Source: three-view drawing plus pictorial views. Frame: mm from the lowest corner of the part. Round coordinates to 2 decimals unless told otherwise and drop trailing zeros. Loops run counter-clockwise (first coordinate to the right, second up) from the corner with the lowest first, then second, coordinate; pieces in that order, holes last. Notation, with made-up numbers: (6, -5) -> (15, -5) arc R8 cw to (15, 8) -> close; hole circle Ø1 at (89, 20). An arc over 180 degrees is marked (long way). Put each result on its own line as item: value. Start each with the question number.
1. Cut plane B-B (y = 52.5). Return the cut outline in (x, z).
2. Cut plane C-C (z = 3.3). State how many separate pieces and enclosed holes the cut face has, then the cut area to 3 significant figures.
3. Cut plane D-D (y = 43). Return the cut outline in (x, z), then the cut area to 3 significant figures.
4. Material intervals for L1, parallel to X at y = 59, z = 1.5; L2, parallel to X at y = 62.5, z = 2.25; L3, parallel to Y at x = 12, z = 1.75, sorted ascending.
5. Cut plane A-A (x = 12). Return the cut outline in (y, z), then the cut area to 3 significant figures.
6. Contact query for flat-ended pins moving along their axis: pin 1 (2 mm diameter, centred on y = 63, z = 2, fed in from -X); pin 2 (1.2 mm diameter, centred on x = 9.5, z = 2.5, fed in from -Y); pin 3 (2 mm diameter, centred on y = 61.5, z = 1.5, fed in from +X); pin 4 (1.2 mm diameter, centred on x = 63, z = 2, fed in from +Y). Output: stop coordinate, or through.
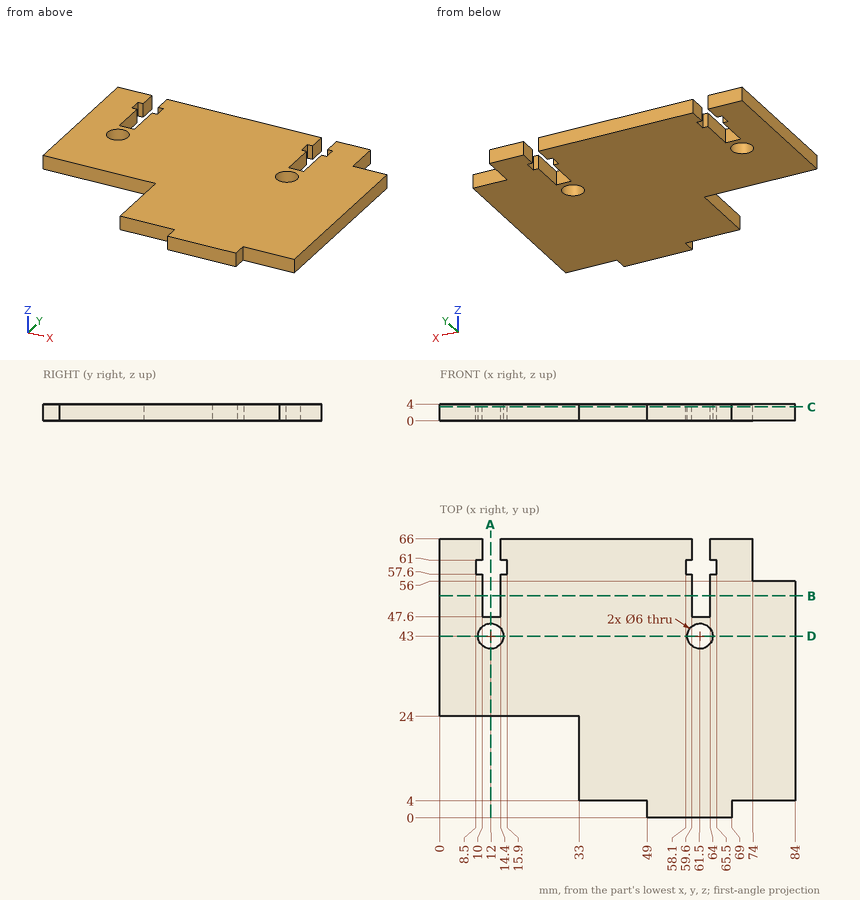
Solution:
1. outline: (0, 0) -> (10, 0) -> (10, 4) -> (0, 4) -> close; (14.4, 0) -> (59.6, 0) -> (59.6, 4) -> (14.4, 4) -> close; (64, 0) -> (84, 0) -> (84, 4) -> (64, 4) -> close
2. separate pieces: 1
2. enclosed holes: 2
2. area: 4,290 mm^2
3. outline: (0, 0) -> (9, 0) -> (9, 4) -> (0, 4) -> close; (15, 0) -> (58.5, 0) -> (58.5, 4) -> (15, 4) -> close; (64.5, 0) -> (84, 0) -> (84, 4) -> (64.5, 4) -> close
3. area: 288 mm^2
4. L1: x = 0 to 8.5, 15.9 to 58.1, 65.5 to 74
4. L2: x = 0 to 10, 14.4 to 59.6, 64 to 74
4. L3: y = 24 to 40, 46 to 47.6
5. outline: (24, 0) -> (40, 0) -> (40, 4) -> (24, 4) -> close; (46, 0) -> (47.6, 0) -> (47.6, 4) -> (46, 4) -> close
5. area: 70.4 mm^2
6. pin 1: stops at x = 0
6. pin 2: stops at y = 24
6. pin 3: stops at x = 74
6. pin 4: stops at y = 47.6
